```python
from build123d import *

# Parameters (mm, degrees)
BOSS_EXTRUDE1_DEPTH = 19.05
SKETCH2_R           = 6.35
CUT_EXTRUDE1_DEPTH  = 2.54
SKETCH3_R           = 6.35
CUT_EXTRUDE2_DEPTH  = 2.54


with BuildPart() as part:
    # Sketch1 → Boss-Extrude1 (new body)
    with BuildSketch(Plane(origin=(0, 0, 0), x_dir=(1, 0, 0), z_dir=(0, 1, 0))):
        Polygon((0, 0), (688.975, 0), (688.975, 241.3), (646.1125, 241.3), (646.1125, 285.75), (42.8625, 285.75), (42.8625, 241.3), (0, 241.3), align=None)
    extrude(amount=BOSS_EXTRUDE1_DEPTH)

    # Sketch2 → Cut-Extrude1 (cut)
    with BuildSketch(Plane(origin=(0, 19.05, 0), x_dir=(1, 0, 0), z_dir=(0, 1, 0))):
        with Locations((555.625, 85.725)):
            Circle(SKETCH2_R)
    extrude(amount=-CUT_EXTRUDE1_DEPTH, mode=Mode.SUBTRACT)

    # Sketch3 → Cut-Extrude2 (cut)
    with BuildSketch(Plane(origin=(0, 19.05, 0), x_dir=(1, 0, 0), z_dir=(0, 1, 0))):
        with Locations((314.325, 34.925)):
            Circle(SKETCH3_R)
    extrude(amount=-CUT_EXTRUDE2_DEPTH, mode=Mode.SUBTRACT)


solid = part.part
```
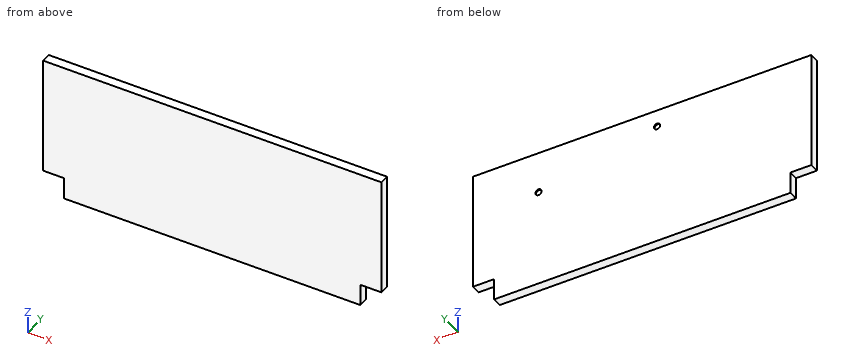
Part model, mm, in its own coordinate system. Coordinates: 2 decimals unless noted, no trailing zeros. Loops run counter-clockwise (first coordinate to the right, second up) from the corner with the lowest first, then second, coordinate; pieces in that order, holes last. Notation, with made-up numbers: (-8, -40) - (14, -40) arc R8 cw to (14, -34) - close; hole circle Ø5 at (-23.75, 22). An arc over 180 degrees is marked (long way). Write item = value, one per line. Start each with the question number.
Item 1: Flat gauge pins, fed straight in: pin 1 Ø5.5 at (y, z) = (11.5, -258.5) entering from -X; pin 2 Ø9.5 at (y, z) = (5.5, -268) entering from +X; pin 3 Ø6 at (x, z) = (114.5, -229) entering from -Y; pin 4 Ø10 at (x, z) = (314.5, -35.5) entering from +Y. Where does each tip first touch, or does it go through?
Item 2: Wall check: L1, parallel to X at y = 14.25, z = -256.5; L2, parallel to Z at x = 649, y = 11.25. Give the ranges that are in metal, low to high. Write a range as from..to.
Item 3: Cut at B-B, the plane z = -248.5. Give the cut face in (x, y).
The answers:
q1.pin_1 = 42.86
q1.pin_2 = 646.11
q1.pin_3 = 0
q1.pin_4 = 16.51
q2.L1 = 42.86..646.11
q2.L2 = -241.3..0
q3.outline = (42.86, 0) - (646.11, 0) - (646.11, 19.05) - (42.86, 19.05) - close
